from build123d import *

# Parameters (mm, degrees)
SKETCH_1_R      = 3
EXTRUDE_1_DEPTH = 8.2
SKETCH_3_R      = 2.9
SKETCH_4_R      = 4
EXTRUDE_2_DEPTH = 4


with BuildPart() as part:
    # ｽｹｯﾁ1 → ﾎﾞｽ - 押し出し1 (new body)
    with BuildSketch(Plane.XY):
        Circle(SKETCH_1_R)
    extrude(amount=EXTRUDE_1_DEPTH)

    # ｽｲｰﾌﾟ1: sweep along a path in ｽｹｯﾁ2
    with BuildLine(Plane(origin=(0, 0, 0), x_dir=(0, 0, -1), z_dir=(1, 0, 0))) as sweep_1_path:
        CenterArc((-18.3, 0), 10.1, 0, 360)
    # ｽｹｯﾁ3 → ｽｲｰﾌﾟ1 (sweep)
    with BuildSketch(Plane(origin=(0, 0, 0), x_dir=(1, 0, 0), z_dir=(0, 1, 0))):
        with Locations((0, -8.2)):
            Circle(SKETCH_3_R)
    sweep(path=sweep_1_path.line)

    # ｽｹｯﾁ4 → ﾎﾞｽ - 押し出し2 (add)
    with BuildSketch(Plane.XY.offset(8.2)):
        Circle(SKETCH_4_R)
    extrude(amount=-EXTRUDE_2_DEPTH)


solid = part.part
The model under review builds one solid part; all positions refer to its coordinate system, in mm. Round coordinates to 2 decimals unless told otherwise and drop trailing zeros. Loops run counter-clockwise (first coordinate to the right, second up) from the corner with the lowest first, then second, coordinate; pieces in that order, holes last. Notation, with made-up numbers: M 14.5,-6.75 L 42.5,-6.75 A31 ccw 42.5,23.25 Z; hole C 20,-21 d10. An arc over 180 degrees is marked long. Answer as a JSON object with one key per item and string values.
Item 1: We need section A-A, the plane y = 0. State the section outline as (x, z) points, and give its area (3 significant figures).
Check sheet entries:
{"outline": "M -4,4.2 L -3,4.2 L -3,0 L 3,0 L 3,4.2 L 4,4.2 L 4,8.2 L 2.9,8.2 A2.9 ccw -2.9,8.2 L -4,8.2 Z; C 0,28.4 d5.8", "area": "96.8 mm2"}
Item 2: The part is to be moulded in two halves that separate along Y. For faces 1 (the face through (0, 0, 0)), 2 (the face through (-3, 0, 2)), say which applies: +Y half, -Y half, draft (parallel to the pull), parting line (faces both ways), or undercut.
Check sheet entries:
{"face 1": "draft", "face 2": "parting line"}
Item 3: We need section B-B, the plane x = 0. State the section outline as (y, z) points.
Check sheet entries:
{"outline": "M -4,4.2 L -3,4.2 L -3,0 L 3,0 L 3,4.2 L 4,4.2 L 4,5.93 A13 ccw long -4,5.93 Z; hole C 0,18.3 d14.4"}
Item 4: For line 1 along Y through (x, z) = (1, 17.5); line 2 along X through (y, z) = (-7.75, 25); line 3 along Y through (x, z) = (0, 21), list the stretches that pass through material, from the lowest coordinate up.
Check sheet entries:
{"line 1": "-12.8 to -7.33, 7.33 to 12.8", "line 2": "-2.9 to 2.9", "line 3": "-12.72 to -6.67, 6.67 to 12.72"}
Item 5: We need section C-C, the plane x = 1.5. State the section outline as (y, z) points, and give its area (3 significant figures).
Check sheet entries:
{"outline": "M -3.71,4.2 L -2.6,4.2 L -2.6,0 L 2.6,0 L 2.6,4.2 L 3.71,4.2 L 3.71,6.28 A12.58 ccw long -3.71,6.28 Z; hole C 0,18.3 d15.24", "area": "349 mm2"}
Item 6: Clearance check with flat-ended pins moving along their axes: P1, Ø1, axis at x = 0, z = 20, coming from the -Y side; P2, Ø1.5, axis at y = -5.5, z = 4, coming from the +X side; P3, Ø0.6, axis at x = -3.5, y = 0, coming from the +Z side; P4, Ø5, axis at y = -4.5, z = 21, coming from the +X side. State where each tip first meets the part, or that it passes through.
Check sheet entries:
{"P1": "y = -12.94", "P2": "through", "P3": "z = 8.2", "P4": "x = 1.7"}
